For this review, take the finished solid that the model builds, in its own axes (mm). Face numbers are marked on the shaded views. A direction names the side the tool comes from. Round coordinates to 2 decimals unless told otherwise and drop trailing zeros. Loops run counter-clockwise (first coordinate to the right, second up) from the corner with the lowest first, then second, coordinate; pieces in that order, holes last.
1. Draft analysis for pull direction X (two halves, no side actions). For the marked faces 1, 2 and 3, state which applies: released by +X, released by -X, zero draft, split by the parting line, or undercut.
2. To check wall thickness, follow line 1 along X through (y, z) = (4.75, -2.5); line 2 along Z through (x, y) = (15.5, 7.25); line 3 along Z through (x, y) = (82.5, 0). State the ranges of each line that lie inside material, in increasing order.
3. Consider section A-A on x = 9. State the section outline as (y, z) points (3 decimals), then the cut area to 3 significant figures.
4. Clearance check with flat-ended pins moving along their axes: pin 1 Ø6.5 at (y, z) = (0, 22.225) entering from +X; pin 2 Ø5.5 at (y, z) = (0, -12.7) entering from -X; pin 3 Ø3 at (x, y) = (-32.5, -4) entering from -Z; pin 4 Ø5.5 at (y, z) = (2.5, 7.5) entering from -X. State where each tip first meets the part, or that it passes through.
5. Consider section D-D on z = -21. State the section outline as (x, y) points (3 decimals), then the cut area to 3 significant figures.
6. Tool access review of the marked faces 4, 5, 6 and 7: name each direction out of +Z, -Z, +X, -X, +Y, -Y from which nothing blocks a thin tool from reaching the whole face with its end or side.
7. Consider section B-B on z = 6.35. State the section outline as (x, y) points (3 decimals), then the cut area to 3 significant figures.
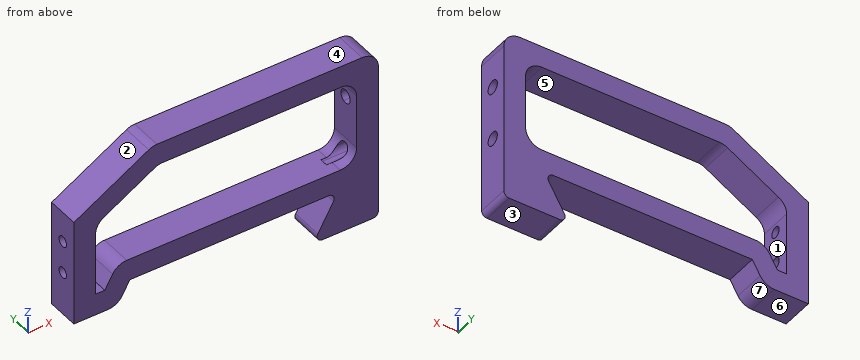
from build123d import *

# Parameters (mm, degrees)
F1_DEPTH      = 9.525
F1_DEPTH_BACK = 9.525
F2_R          = 9.525
F3_R          = 3.175
F4_R          = 3.175
F5_DEPTH      = 12.7
F7_DEPTH      = 25.4


with BuildPart() as f1:
    # F0 (on Front) → F1 (new body, two sides)
    with BuildSketch(Plane.XZ) as f1_sk:
        Polygon((-42.952364, 50.8), (-88.9, 24.27212), (-88.9, -38.1), (-63.5, -38.1), (-56.167652, -25.4), (65.464697, -25.4), (50.8, -50.8), (88.9, -50.8), (88.9, 50.8), align=None)
        Polygon((-39.549409, 38.1), (76.2, 38.1), (76.2, -12.7), (-63.5, -12.7), (-70.832348, -25.4), (-76.2, -25.4), (-76.2, 16.939772), align=None, mode=Mode.SUBTRACT)
    extrude(amount=F1_DEPTH)
    extrude(f1_sk.sketch, amount=-F1_DEPTH_BACK)

    # F2
    f2_edges = [f1.edges().sort_by_distance(p)[0] for p in [
        (88.9, 0, 50.8),
        (-42.952364, 0, 50.8),
        (-63.5, 0, -38.1),
        (-76.2, 0, 16.939772),
        (-39.549409, 0, 38.1),
        (76.2, 0, 38.1),
        (-63.5, 0, -12.7),
        (76.2, 0, -12.7),
    ]]
    fillet(f2_edges, radius=F2_R)

    # F3
    f3_edges = [f1.edges().sort_by_distance(p)[0] for p in [
        (50.8, 0, -50.8),
        (65.464697, 0, -25.4),
        (88.9, 0, -50.8),
    ]]
    fillet(f3_edges, radius=F3_R)

    # F4 (on face) → F5 (cut, through all)
    with BuildSketch(Plane(origin=(-88.9, 0, 0), x_dir=(0, -1, 0), z_dir=(-1, 0, 0))):
        with Locations((0, -12.7)):
            Circle(F4_R)
        with Locations((0, 6.35)):
            Circle(F4_R)
    extrude(amount=-F5_DEPTH, mode=Mode.SUBTRACT)

    # F6 (on face) → F7 (cut)
    with BuildSketch(Plane.YZ.offset(88.9)):
        with BuildLine():
            Line((1.5875, -13.162419), (1.5875, -5.887581))
            ThreePointArc((1.5875, -5.887581), (-3.96875, -9.525), (1.5875, -13.162419))
        make_face()
        with BuildLine():
            ThreePointArc((3.96875, -9.525), (3.320494, -7.351226), (1.5875, -5.887581))
            Line((1.5875, -5.887581), (1.5875, -13.162419))
            ThreePointArc((1.5875, -13.162419), (3.320494, -11.698774), (3.96875, -9.525))
        make_face()
        with BuildLine():
            ThreePointArc((1.5875, 18.587581), (3.320494, 20.051226), (3.96875, 22.225))
            ThreePointArc((3.96875, 22.225), (3.320494, 24.398774), (1.5875, 25.862419))
            Line((1.5875, 25.862419), (1.5875, 18.587581))
        make_face()
        with BuildLine():
            Line((1.5875, 18.587581), (1.5875, 25.862419))
            ThreePointArc((1.5875, 25.862419), (-3.96875, 22.225), (1.5875, 18.587581))
        make_face()
    extrude(amount=-F7_DEPTH, mode=Mode.SUBTRACT)


solid = f1.part
Resolved:
1. face 1: undercut
1. face 2: released by -X
1. face 3: zero draft
2. line 1: x = -88.9 to -76.2, 76.2 to 88.9
2. line 2: z = -25.4 to -12.7, 38.1 to 50.8
2. line 3: z = -50.8 to -13.49, -5.56 to 18.26, 26.19 to 50.27
3. outline: (-9.525, -25.4) - (9.525, -25.4) - (9.525, -12.7) - (-9.525, -12.7) - close; (-9.525, 38.1) - (9.525, 38.1) - (9.525, 50.8) - (-9.525, 50.8) - close
3. area: 484 mm2
4. pin 1: stops at x = -61.42
4. pin 2: stops at x = -64.7
4. pin 3: stops at z = -25.4
4. pin 4: stops at x = -88.9
5. outline: (-88.9, -9.525) - (-76.2, -9.525) - (-76.2, 9.525) - (-88.9, 9.525) - close; (-68.292, -9.525) - (88.9, -9.525) - (88.9, 9.525) - (-68.292, 9.525) - close
5. area: 3,240 mm2
6. face 4: +Z, +X, -X, +Y, -Y
6. face 5: +Y, -Y
6. face 6: -Z, -X, +Y, -Y
6. face 7: -Z, +Y, -Y
7. outline: (-88.9, -9.525) - (-76.2, -9.525) - (-76.2, -3.175) - (-88.9, -3.175) - close; (-88.9, 3.175) - (-76.2, 3.175) - (-76.2, 9.525) - (-88.9, 9.525) - close; (76.2, -9.525) - (88.9, -9.525) - (88.9, 9.525) - (76.2, 9.525) - close
7. area: 403 mm2
